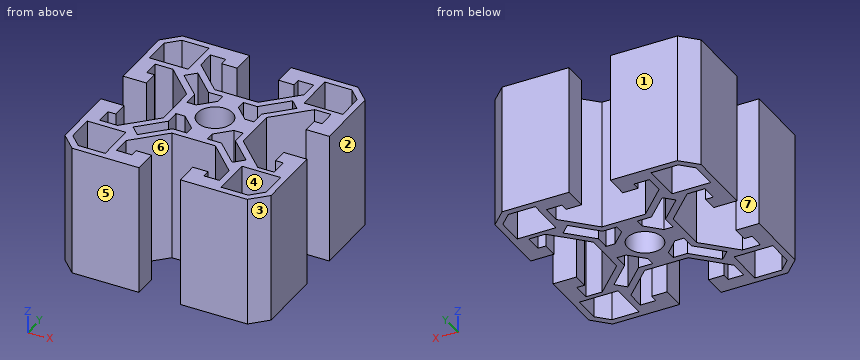
```python
from build123d import *

# Parameters (mm, degrees)
SKETCH1_R      = 3.4
EXTRUDE1_DEPTH = 25.4


with BuildPart() as part:
    # Sketch1 → Extrude1 (new body)
    with BuildSketch(Plane.XY):
        Polygon((4.225, 7.75), (-4.225, 7.75), (-10, 13.525), (-10, 17), (-7, 17), (-7, 15.5), (-4, 15.5), (-4, 20), (-17, 20), (-20, 17), (-20, 4.0635), (-15.5, 4.0635), (-15.5, 7), (-17, 7), (-17, 10), (-13.525, 10), (-7.75, 4.225), (-7.75, -4.225), (-13.525, -10), (-17, -10), (-17, -7), (-15.5, -7), (-15.5, -4), (-20, -4), (-20, -17), (-17, -20), (-4, -20), (-4, -15.5), (-7, -15.5), (-7, -17), (-10, -17), (-10, -13.525), (-4.225, -7.75), (4.225, -7.75), (10, -13.525), (10, -17), (7, -17), (7, -15.5), (4, -15.5), (4, -20), (17, -20), (20, -17), (20, -4.0635), (15.5, -4.0635), (15.5, -7), (17, -7), (17, -10.2921), (13.8171, -10.2921), (7.75, -4.225), (7.75, 4.225), (13.8171, 10.2921), (17, 10.2921), (17, 7), (15.5, 7), (15.5, 4.0635), (20, 4.0635), (20, 17), (17, 20), (4, 20), (4, 15.5), (7, 15.5), (7, 17), (10, 17), (10, 13.525), align=None)
        Circle(SKETCH1_R, mode=Mode.SUBTRACT)
        Polygon((-18.75, -16.482233), (-16.482233, -18.75), (-11.25, -18.75), (-11.25, -11.25), (-18.75, -11.25), align=None, mode=Mode.SUBTRACT)
        Polygon((18.75, 16.482233), (16.482233, 18.75), (11.25, 18.75), (11.25, 11.25), (18.75, 11.25), align=None, mode=Mode.SUBTRACT)
        Polygon((2, -6.5), (4.742767, -6.5), (9.197655, -10.954888), (10.954888, -9.197655), (6.5, -4.742767), (6.5, -2), (4.745788, -2), (2, -4.745788), align=None, mode=Mode.SUBTRACT)
        Polygon((6.5, 2), (6.5, 4.742767), (10.954888, 9.197655), (9.197655, 10.954888), (4.742767, 6.5), (2, 6.5), (2, 4.745788), (4.745788, 2), align=None, mode=Mode.SUBTRACT)
        Polygon((-2, 6.5), (-4.742767, 6.5), (-9.197655, 10.954888), (-10.954888, 9.197655), (-6.5, 4.742767), (-6.5, 2), (-4.745788, 2), (-2, 4.745788), align=None, mode=Mode.SUBTRACT)
        Polygon((-6.5, -2), (-6.5, -4.742767), (-10.954888, -9.197655), (-9.197655, -10.954888), (-4.742767, -6.5), (-2, -6.5), (-2, -4.745788), (-4.745788, -2), align=None, mode=Mode.SUBTRACT)
        Polygon((-16.482233, 18.75), (-18.75, 16.482233), (-18.75, 11.25), (-11.25, 11.25), (-11.25, 18.75), align=None, mode=Mode.SUBTRACT)
        Polygon((16.482233, -18.75), (18.75, -16.482233), (18.75, -11.25), (11.25, -11.25), (11.25, -18.75), align=None, mode=Mode.SUBTRACT)
    extrude(amount=EXTRUDE1_DEPTH)


solid = part.part
```
Here's how the part is built. I have some questions about the finished solid (model axes, mm). Face numbers are marked on the shaded views. A direction names the side the tool comes from. Give positions to 0.01 mm unless a question says otherwise; leave off trailing zeros. Order: outer loops, then holes, each group sorted by start corner. A loop starts at its lowest first (then second) coordinate and runs counter-clockwise, first axis right, second up. Notation, with made-up numbers: (50.25, 84) -> (66.25, 84) arc R24 ccw to (66.25, 95) -> close; hole circle Ø11 at (-38, 55.25). An arc over 180 degrees is marked (long way). Use CSV: the item, a comma, the result in double quotes. Start each with the question number.
Item 1: I'm going to push flat-ended pins straight in: P1, Ø6, axis at x = 0.5, y = -11, coming from the +Z side; P2, Ø4, axis at y = 1.5, z = 15, coming from the -X side. Where does each tip first touch, or does it pass through?
Item 2: If I drill on probe 1 along Y at (x, z) = (-14.5, 16.5); probe 2 along Y at (x, z) = (15, 14.25); probe 3 along Y at (x, z) = (0, 9.75), over which ranges is the centre line in solid material (lowest first)? Write a range as [from, to].
Item 3: Thinking about a two-plate mould opening in Y: for the marked faces 1, 2, 3 and 4, which applies, pulls with the +Y half, pulls with the -Y half, needs draft (parallel to the pull), parting line crosses it, or undercut?
Item 4: Suppose I cut it at C-C (x = 13). List the corners of the cut face in (y, z) for me (3 decimals), and give its area (3 significant figures).
Item 5: Suppose I cut it at A-A (y = 0). List the corners of the cut face in (x, z) for me.
Item 6: On a 3-axis mill with a long thin cutter (end or side, diameter ignored), from which of +Z, -Z, +X, -X, +Y, -Y can I reach the whole of each face in a straight line? I mean the marked faces 5, 6 and 7. Say none if no direction works.
Answer block:
1,P1,"passes through"
1,P2,"stops at x = -7.75"
2,probe 1,"y = [-20, -18.75], [-11.25, -10], [10, 11.25], [18.75, 20]"
2,probe 2,"y = [-20, -18.75], [-11.25, -10.29], [10.29, 11.25], [18.75, 20]"
2,probe 3,"y = [-7.75, -3.4], [3.4, 7.75]"
3,face 1,"pulls with the +Y half"
3,face 2,"needs draft"
3,face 3,"pulls with the -Y half"
3,face 4,"undercut"
4,outline,"(-20, 0) -> (-18.75, 0) -> (-18.75, 25.4) -> (-20, 25.4) -> close; (-11.25, 0) -> (-9.475, 0) -> (-9.475, 25.4) -> (-11.25, 25.4) -> close; (9.475, 0) -> (11.25, 0) -> (11.25, 25.4) -> (9.475, 25.4) -> close; (18.75, 0) -> (20, 0) -> (20, 25.4) -> (18.75, 25.4) -> close"
4,area,"154 mm^2"
5,outline,"(-7.75, 0) -> (-3.4, 0) -> (-3.4, 25.4) -> (-7.75, 25.4) -> close; (3.4, 0) -> (7.75, 0) -> (7.75, 25.4) -> (3.4, 25.4) -> close"
6,face 5,"+Z, -Z, +X, -X, -Y"
6,face 6,"+Z, -Z"
6,face 7,"+Z, -Z, -X"
